```python
from build123d import *

# Parameters (mm, degrees)
IZIM6_R                     = 42.5
IZIM6_R_2                   = 38
Y_KSEKLIK_EKSTR_ZYON1_DEPTH = 40
IZIM7_R                     = 42.5
Y_KSEKLIK_EKSTR_ZYON2_DEPTH = 5
IZIM8_R                     = 2
IZIM8_R_2                   = 6.25
KES_EKSTR_ZYON2_DEPTH       = 5
KES_EKSTR_ZYON4_DEPTH       = 5


with BuildPart() as part:
    # Çizim6 → Yükseklik-Ekstrüzyon1 (new body)
    with BuildSketch(Plane(origin=(0, 0, 0), x_dir=(1, 0, 0), z_dir=(0, 1, 0))):
        with Locations(Location((0, 0, 0), (0, 0, 270))):
            Circle(IZIM6_R)
        with Locations(Location((0, 0, 0), (0, 0, 270))):
            Circle(IZIM6_R_2, mode=Mode.SUBTRACT)
    extrude(amount=Y_KSEKLIK_EKSTR_ZYON1_DEPTH)

    # Çizim7 → Yükseklik-Ekstrüzyon2 (add)
    with BuildSketch(Plane(origin=(0, 40, 0), x_dir=(1, 0, 0), z_dir=(0, 1, 0))):
        with Locations(Location((0, 0, 0), (0, 0, 270))):
            Circle(IZIM7_R)
    extrude(amount=Y_KSEKLIK_EKSTR_ZYON2_DEPTH)

    # Çizim8 → Kes-Ekstrüzyon2 (cut)
    with BuildSketch(Plane(origin=(0, 45, 0), x_dir=(1, 0, 0), z_dir=(0, 1, 0))):
        with Locations(Location((0, 32.5, 0), (0, 0, 270))):
            Circle(IZIM8_R)
        with Locations(Location((-32.5, 0, 0), (0, 0, 270))):
            Circle(IZIM8_R)
        with Locations(Location((32.5, 0, 0), (0, 0, 270))):
            Circle(IZIM8_R)
        with Locations(Location((0, -32.5, 0), (0, 0, 270))):
            Circle(IZIM8_R)
        with Locations(Location((0, 0, 0), (0, 0, 270))):
            Circle(IZIM8_R_2)
        with Locations(Location((-15.5, 6, 0), (0, 0, 270))):
            Circle(IZIM8_R)
        with Locations(Location((-7.75, 19.423393759, 0), (0, 0, 270))):
            Circle(IZIM8_R)
        with Locations(Location((7.75, 19.423393759, 0), (0, 0, 270))):
            Circle(IZIM8_R)
        with Locations(Location((15.5, 6, 0), (0, 0, 270))):
            Circle(IZIM8_R)
        with Locations(Location((7.75, -7.423393759, 0), (0, 0, 270))):
            Circle(IZIM8_R)
        with Locations(Location((-7.75, -7.423393759, 0), (0, 0, 270))):
            Circle(IZIM8_R)
    extrude(amount=-KES_EKSTR_ZYON2_DEPTH, mode=Mode.SUBTRACT)

    # Çizim11 → Kes-Ekstrüzyon4 (cut)
    with BuildSketch(Plane(origin=(0, 45, 0), x_dir=(1, 0, 0), z_dir=(0, 1, 0))):
        with BuildLine():
            Line((-33.71988341, 7.295167084), (-29.810331711, 6.44935061))
            ThreePointArc((-29.810331711, 6.44935061), (-22.597803721, 20.483878221), (-9.336800782, 29.035739205))
            Line((-9.336800782, 29.035739205), (-10.561299245, 32.843705002))
            ThreePointArc((-10.561299245, 32.843705002), (-25.561450111, 23.170288479), (-33.71988341, 7.295167084))
        make_face()
    extrude(amount=-KES_EKSTR_ZYON4_DEPTH, mode=Mode.SUBTRACT)


solid = part.part
```
Could you check a few things on this model? Use its own coordinates, in mm. A direction names the side the tool comes from. Give positions to 0.01 mm unless a question says otherwise; leave off trailing zeros. Write each loop counter-clockwise with the first axis right and the second up, starting at its lowest first coordinate (ties: lowest second). Pieces come first, ordered by that corner, then holes. Notation, with made-up numbers: (66.25, 66.25) - (101.25, 66.25) arc R28 ccw to (101.25, 99.25) - close; hole circle Ø5 at (-25, 33.5). An arc over 180 degrees is marked (long way). One line per item, written item: value. Start each with the question number.
Item 1: If we mould it in two halves opening along X, with no side actions, what happens to faces 1 (the face through (-0.766, 42.535, 34.347)), 2 (the face through (-25.861, 22.185, -33.727)), 3 (the face through (1, 45, 9))? For each: +X half, -X half, draft (parallel to the pull), parting line (faces both ways), or undercut.
Item 2: Please list where these lines run through material, in increasing order: line 1 (X direction, y = 43.2, z = 0); line 2 (Y direction, x = 1, z = 22.5); line 3 (X direction, y = 5, z = 4.5). Write a range as from..to.
Item 3: Imagine slicing it at A-A, the plane x = 0. List the corners of the cut face in (y, z) for me.
Item 4: Imagine slicing it at C-C, the plane z = -0.5. List the corners of the cut face in (x, y) for me.
Item 5: Which directions (+Z, -Z, +X, -X, +Y, -Y) give clear straight access to the entire face, cutting with the end or side of a thin tool? Please do faces 4 (the face through (-22, 0, -32)), 5 (the face through (-23.122, 19.72, -30.156)), 6 (the face through (-9.94, 42.54, -30.91)).
Item 6: I'm going to push flat-ended pins straight in: pin 1 (4 mm diameter, centred on y = 18, z = 30, fed in from -X); pin 2 (1 mm diameter, centred on y = 28, z = -27, fed in from +X); pin 3 (4.5 mm diameter, centred on x = 15.5, z = -6, fed in from -Y). Where does each tip first touch, or does it pass through?
Item 7: Imagine slicing it at D-D, the plane x = 32.5. List the corners of the cut face in (y, z) for me.
Item 8: Imagine slicing it at B-B, the plane z = 32.5. List the corners of the cut face in (x, y) for me.
Geometry says:
1. face 1: undercut
1. face 2: parting line
1. face 3: draft
2. line 1: -42.5..-34.5, -30.5..-6.25, 6.25..30.5, 34.5..42.5
2. line 2: 40..45
2. line 3: -42.26..-37.73, 37.73..42.26
3. outline: (0, -42.5) - (45, -42.5) - (45, -34.5) - (40, -34.5) - (40, -38) - (0, -38) - close; (0, 38) - (40, 38) - (40, 34.5) - (45, 34.5) - (45, 42.5) - (0, 42.5) - close; (40, -30.5) - (45, -30.5) - (45, -6.25) - (40, -6.25) - close; (40, 6.25) - (45, 6.25) - (45, 30.5) - (40, 30.5) - close
4. outline: (-42.5, 0) - (-38, 0) - (-38, 40) - (-34.44, 40) - (-34.44, 45) - (-42.5, 45) - close; (-30.56, 40) - (-6.23, 40) - (-6.23, 45) - (-30.56, 45) - close; (6.23, 40) - (30.56, 40) - (30.56, 45) - (6.23, 45) - close; (34.44, 40) - (38, 40) - (38, 0) - (42.5, 0) - (42.5, 45) - (34.44, 45) - close
5. face 4: +Z, -Z, +X, -X, -Y
5. face 5: -Y
5. face 6: +Y, -Y
6. pin 1: x = -31.97
6. pin 2: x = 33.23
6. pin 3: y = 40
7. outline: (0, -27.39) - (45, -27.39) - (45, -2) - (40, -2) - (40, -19.69) - (0, -19.69) - close; (0, 19.69) - (40, 19.69) - (40, 2) - (45, 2) - (45, 27.39) - (0, 27.39) - close
8. outline: (-27.39, 0) - (-19.69, 0) - (-19.69, 40) - (-2, 40) - (-2, 45) - (-27.39, 45) - close; (2, 40) - (19.69, 40) - (19.69, 0) - (27.39, 0) - (27.39, 45) - (2, 45) - close
